Can you work these out from the model? Positions are in its coordinate system, mm. A direction names the side the tool comes from. Round coordinates to 2 decimals unless told otherwise and drop trailing zeros. Loops run counter-clockwise (first coordinate to the right, second up) from the corner with the lowest first, then second, coordinate; pieces in that order, holes last.
(1) I want a section at B-B on z = 5. Write out the boundary of the cut face in (x, y), plus the area to 3 significant figures.
(2) If I drill on line 1 along Z through (x, y) = (0, 0.9); line 2 along Z through (x, y) = (1, 0); line 3 along Y through (x, z) = (-0.15, 12.5), over which ranges is the centre line in solid material (lowest first)?
(3) Which directions (+Z, -Z, +X, -X, +Y, -Y) give clear straight access to the entire face, cutting with the end or side of a thin tool? Please do faces 4 (the face through (1.5, 2, 21.4)), 5 (the face through (-0.208, 0.028, 18.414)), 6 (the face through (1.5, -2, 21.4)), 7 (the face through (0, 2.4, 9.5)), 8 (the face through (-1.5, -2, 3.6)).
(4) I want a section at D-D on z = 9.25. Write out the boundary of the cut face in (x, y), plus the area to 3 significant figures.
(5) I want a section at C-C on y = 0. Write out the boundary of the cut face in (x, z), plus the area to 3 significant figures.
(6) I want a section at A-A on x = 0. Write out the boundary of the cut face in (y, z), plus the area to 3 significant figures.
(7) Will these pins go through, and if not, where does the flat tip stop? pin 1 Ø1 at (y, z) = (1.5, 17.5) entering from +X; pin 2 Ø2.5 at (x, z) = (0, 20) entering from +Y; pin 3 Ø2 at (y, z) = (-1.5, 2.5) entering from +X; pin 4 Ø2 at (x, z) = (0, 21.5) entering from -Y.
(8) Thinking about a two-plate mould opening in Z: for faces 1 (the face through (-0.35, 0.03, 6.56)), 2 (the face through (-1.5, 2, 3.6)), 3 (the face through (0, 0, 25)), which applies, released by +Z, released by -Z, zero draft, split by the parting line, or undercut?
Autodesk Inventor part; units mm, degrees
ref_plane "YZ Plane" through (0, 0, 0) normal (1, 0, 0) x (0, 1, 0)
ref_plane "XZ Plane" through (0, 0, 0) normal (0, 1, 0) x (-1, 0, 0)
ref_plane "XY Plane" through (0, 0, 0) normal (0, 0, 1) x (1, 0, 0)
sketch "スケッチ1" plane through (0, 0, 0) normal (0, 0, 1) x (1, 0, 0)
  circle A0 centre (0, 0) radius 3
  dimension "d0" = 6
extrude "押し出し1" add sketch "スケッチ1" along normal blind 25
sketch "スケッチ2" plane through (0, 0, 25) normal (0, 0, 1) x (1, 0, 0)
  line L0 (-2.2832, 2) -> (2.2938, 2)
  line L1 (-2.2832, -2) -> (2.3454, -2)
  arc A0 (-2.2361, 2) -> (-2.2361, -2) centre (0, 0) ccw construction
  arc A1 (2.2361, 2) -> (-2.2361, 2) centre (0, 0) ccw
  arc A2 (2.2361, -2) -> (2.2361, 2) centre (0, 0) ccw construction
  arc A3 (-2.2361, -2) -> (2.2361, -2) centre (0, 0) ccw
  dimension "d5" = 2
  dimension "d6" = 6
  dimension "d7" = 2
extrude "押し出し2" cut sketch "スケッチ2" against normal blind 9.5
sketch "スケッチ3" plane through (0, 0, 0) normal (0, 0, -1) x (-1, 0, 0)
  arc A0 (-2.2361, -2) -> (2.2361, -2) centre (0, 0) ccw
  line L0 (-2.2361, 2) -> (2.2361, 2)
  line L1 (-2.2361, -2) -> (2.2361, -2)
  arc A1 (2.2361, -2) -> (2.2361, 2) centre (0, 0) ccw construction
  arc A2 (-2.2361, 2) -> (-2.2361, -2) centre (0, 0) ccw construction
  arc A3 (2.2361, 2) -> (-2.2361, 2) centre (0, 0) ccw
  arc A4 (2.2361, -2) -> (2.2361, 2) centre (0, 0) ccw construction
  dimension "d13" = 2
  dimension "d14" = 2
extrude "押し出し3" cut sketch "スケッチ3" against normal blind 9.5
sketch "スケッチ4" plane through (-2.2361, 2, 0) normal (0, 1, 0) x (1, 0, 0)
  circle A0 centre (2.2361, -5) radius 1.6
  circle A1 centre (2.2361, -20) radius 1.6
  line L0 (0, 0) -> (4.4721, 0)
  point P0 (2.2361, 0)
  point P1 (2.2361, 0)
  point P2 (2.2361, 0)
  dimension "d17" = 3.2
  dimension "d18" = 3.2
  dimension "d19" = 15
  dimension "d20" = 5
extrude "押し出し4" cut sketch "スケッチ4" against normal through all
properties part number "上昇機構_固定軸ベアリングの" material "アルミニウム 6061"
Filled sheet:
1. outline: (-2.24, -2) - (-1.6, -2) - (-1.6, 2) - (-2.24, 2) arc R3 ccw to start; (1.6, -2) - (2.24, -2) arc R3 ccw to (2.24, 2) - (1.6, 2) - close
1. area: 9.28 mm2
2. line 1: z = 0 to 3.4, 6.6 to 18.4, 21.6 to 25
2. line 2: z = 0 to 3.75, 6.25 to 18.75, 21.25 to 25
2. line 3: y = -3 to 3
3. face 4: +Z, +X, -X, +Y
3. face 5: +Y, -Y
3. face 6: +Z, +X, -X, -Y
3. face 7: -Z, +X, -X, +Y
3. face 8: -Z, +X, -X, -Y
4. outline: (-2.24, -2) - (2.24, -2) arc R3 ccw to (2.24, 2) - (-2.24, 2) arc R3 ccw to start
4. area: 22.1 mm2
5. outline: (-3, 0) - (3, 0) - (3, 25) - (-3, 25) - close; hole circle Ø3.2 at (0, 5); hole circle Ø3.2 at (0, 20)
5. area: 134 mm2
6. outline: (-3, 9.5) - (-2, 9.5) - (-2, 6.6) - (2, 6.6) - (2, 9.5) - (3, 9.5) - (3, 15.5) - (2, 15.5) - (2, 18.4) - (-2, 18.4) - (-2, 15.5) - (-3, 15.5) - close; (-2, 0) - (2, 0) - (2, 3.4) - (-2, 3.4) - close; (-2, 21.6) - (2, 21.6) - (2, 25) - (-2, 25) - close
6. area: 86.4 mm2
7. pin 1: stops at x = 2.83
7. pin 2: passes through
7. pin 3: stops at x = 2.96
7. pin 4: stops at y = -2
8. face 1: undercut
8. face 2: zero draft
8. face 3: released by +Z
